Solid Edge part; units mm, degrees
sketch "Sketch1" plane through (0, 0, 24.2) normal (0, 0, 1) x (1, 0, 0)
  line L0 (-11.5, 14.5) -> (7.5, 14.5)
  line L1 (7.5, 14.5) -> (7.5, 0)
  line L2 (7.5, -14.5) -> (7.5, 0)
  line L3 (-11.5, -14.5) -> (7.5, -14.5)
  line L4 (-11.5, -7.5) -> (-11.5, -14.5)
  line L5 (-11.5, -7.5) -> (-7.5, -7.5)
  line L6 (-7.5, -7.5) -> (-7.5, 0)
  line L7 (-7.5, 7.5) -> (-7.5, 0)
  line L8 (-11.5, 7.5) -> (-7.5, 7.5)
  line L9 (-11.5, 7.5) -> (-11.5, 14.5)
extrude "Protrusion1" add sketch "Sketch1" along normal blind 8
sketch "Sketch2" plane through (-11.5, -11, 28.2) normal (-1, 0, 0) x (0, 1, 0)
  line L0 (1.2229, 1.1809) -> (0, 2.4472)
  line L1 (0, 2.4472) -> (-1.2229, 1.1809)
  arc A0 (1.2229, 1.1809) -> (-1.2229, 1.1809) centre (0, 0) cw
  line L2 (23.2229, 1.1809) -> (22, 2.4472)
  line L3 (22, 2.4472) -> (20.7771, 1.1809)
  arc A1 (23.2229, 1.1809) -> (20.7771, 1.1809) centre (22, 0) cw
extrude "Cutout1" cut sketch "Sketch2" against normal through all
sketch "Sketch3" plane through (-2, 0, 24.2) normal (0, 0, -1) x (-1, 0, 0)
  line L0 (-5.8971, 2.25) -> (-5.8971, -2.25)
  line L1 (-5.8971, -2.25) -> (-2, -4.5)
  line L2 (-2, -4.5) -> (1.8971, -2.25)
  line L3 (1.8971, -2.25) -> (1.8971, 2.25)
  line L4 (1.8971, 2.25) -> (-2, 4.5)
  line L5 (-2, 4.5) -> (-5.8971, 2.25)
extrude "Cutout2" cut sketch "Sketch3" against normal through all
properties material "ABS Plastic, medium impact"
For this review, take the finished solid that the model builds, in its own axes (mm). A direction names the side the tool comes from. Coordinates: 2 decimals unless noted, no trailing zeros. Order: outer loops, then holes, each group sorted by start corner. A loop starts at its lowest first (then second) coordinate and runs counter-clockwise, first axis right, second up. Notation, with made-up numbers: (42.25, -27.5) - (94.25, -27.5) arc R15 ccw to (94.25, -6.5) - close; hole circle Ø5 at (41, 78). An arc over 180 degrees is marked (long way). Answer as a JSON object with one key per item and string values. Group by question number.
1. We need section A-A on z = 28.2. State the section outline as (x, y) points.
2. For probe 1 along Y at (x, z) = (-5.75, 28.2); probe 2 along Y at (x, z) = (-8, 29.5); probe 3 along Y at (x, z) = (-2.75, 28.2), list the stretches that pass through material, from the lowest coordinate up.
3. We need section D-D on x = 3. State the section outline as (y, z) points.
4. We need section B-B on y = 0.5. State the section outline as (x, z) points.
5. For faces 1 (the flat face through (3.897, 0, 28)), 2 (the flat face through (-10, -7.5, 28)), 3 (the flat face through (7.5, 0, 28)), 4 (the flat face through (-2.133, 10.397, 26.377)), list the 3-axis set-ups (+Z, -Z, +X, -X, +Y, -Y) from which the entire face can be reached by the end or side of a thin tool; tool diameter is ignored.
6. Clearance check with flat-ended pins moving along their axes: P1, Ø1.5, axis at x = -8.5, y = 4.5, coming from the +Z side; P2, Ø2, axis at y = -1, z = 28, coming from the -X side. State where each tip first meets the part, or that it passes through.
7. The part is to be moulded in two halves that separate along Z. For faces 5 (the flat face through (-4, 3, 32.2)), 6 (the cylindrical face through (-2.13, 10.94, 29.9)), 7 (the flat face through (-2, -14.5, 28)), 8 (the flat face through (-4, 3, 24.2)), say which applies: pulls with the +Z half, pulls with the -Z half, needs draft (parallel to the pull), parting line crosses it, or undercut.
8. We need section C-C on x = -10. State the section outline as (y, z) points.
Final values:
{
 "1": {"outline": "(-11.5, -14.5) - (7.5, -14.5) - (7.5, -12.7) - (-11.5, -12.7) - close; (-11.5, -9.3) - (7.5, -9.3) - (7.5, 9.3) - (-11.5, 9.3) - (-11.5, 7.5) - (-7.5, 7.5) - (-7.5, -7.5) - (-11.5, -7.5) - close; (-11.5, 12.7) - (7.5, 12.7) - (7.5, 14.5) - (-11.5, 14.5) - close; hole (-3.9, -2.25) - (0, -4.5) - (3.9, -2.25) - (3.9, 2.25) - (0, 4.5) - (-3.9, 2.25) - close"},
 "2": {"probe 1": "-14.5 to -12.7, -9.3 to 9.3, 12.7 to 14.5", "probe 2": "-14.5 to -12.1, -9.9 to -7.5, 7.5 to 9.9, 12.1 to 14.5", "probe 3": "-14.5 to -12.7, -9.3 to -2.91, 2.91 to 9.3, 12.7 to 14.5"},
 "3": {"outline": "(-14.5, 24.2) - (-2.77, 24.2) - (-2.77, 32.2) - (-14.5, 32.2) - close; (2.77, 24.2) - (14.5, 24.2) - (14.5, 32.2) - (2.77, 32.2) - close; hole (-12.22, 27.02) - (-11, 25.75) - (-9.78, 27.02) arc R1.7 ccw (long way) to start; hole (9.78, 27.02) - (11, 25.75) - (12.22, 27.02) arc R1.7 ccw (long way) to start"},
 "4": {"outline": "(-7.5, 24.2) - (-3.9, 24.2) - (-3.9, 32.2) - (-7.5, 32.2) - close; (3.9, 24.2) - (7.5, 24.2) - (7.5, 32.2) - (3.9, 32.2) - close"},
 "5": {"face 1": "+Z, -Z", "face 2": "+Z, -Z, -X", "face 3": "+Z, -Z, +X, +Y, -Y", "face 4": "+X, -X"},
 "6": {"P1": "through", "P2": "x = -7.5"},
 "7": {"face 5": "pulls with the +Z half", "face 6": "undercut", "face 7": "needs draft", "face 8": "pulls with the -Z half"},
 "8": {"outline": "(-14.5, 24.2) - (-7.5, 24.2) - (-7.5, 32.2) - (-14.5, 32.2) - close; (7.5, 24.2) - (14.5, 24.2) - (14.5, 32.2) - (7.5, 32.2) - close; hole (-12.22, 27.02) - (-11, 25.75) - (-9.78, 27.02) arc R1.7 ccw (long way) to start; hole (9.78, 27.02) - (11, 25.75) - (12.22, 27.02) arc R1.7 ccw (long way) to start"}
}
